Read the model definition and answer for the solid it produces. Units are mm, in the model's axes. A direction names the side the tool comes from. Round coordinates to 2 decimals unless told otherwise and drop trailing zeros. Write each loop counter-clockwise with the first axis right and the second up, starting at its lowest first coordinate (ties: lowest second). Pieces come first, ordered by that corner, then holes. Notation, with made-up numbers: (88.25, -19) - (100.25, -19) arc R22 cw to (100.25, 19) - close; hole circle Ø6 at (-29.5, -22). An arc over 180 degrees is marked (long way). Answer as CSV lines item,"result". Start each with the question number.
1) Consider line 1 along X through (y, z) = (8, 2.85); line 2 along Y through (x, z) = (-43, 1.35); line 3 along Z through (x, y) = (-38.75, -10). Determine where each line is inside the solid, lowest interval first.
2) Which of the six approach directions +Z, -Z, +X, -X, +Y, -Y give full straight-line access (tool end or side, diameter ignored) to faces 3 (the cylindrical face through (45.3, 9.2, 1.4)), 4 (the flat face through (-37.54, -10, 2)), 5 (the flat face through (-43.04, -9, 3)), 6 (the flat face through (-1, 0, 4))?
3) Find section A-A on y = -10. Determine the outline of the cut face in (x, z), then the cut area to 3 significant figures.
4) For a pull along Y with two mould halves and no side action, classify faces 1 (the flat face through (-47.54, 0, 2)), 2 (the flat face through (-40.04, 11, 3)) as +Y half, -Y half, draft (parallel to the pull), parting line (faces both ways), or undercut.
5) Each of these flat-tipped pins is pushed along its axis until it touches: pin 1 (1.5 mm diameter, centred on x = -42, z = 2.5, fed in from -Y); pin 2 (1.2 mm diameter, centred on y = -10, z = 2, fed in from -X); pin 3 (1.6 mm diameter, centred on y = 10, z = 2, fed in from +X). Where does it stop, or does it pass through?
from build123d import *

# Parameters (mm, degrees)
ESQUISSE1_W             = 95.08
ESQUISSE1_H             = 33.02
ESQUISSE1_W_2           = 3
ESQUISSE1_H_2           = 6
BOSS_EXTRU_1_DEPTH      = 4
CONG_1_R                = 3
ESQUISSE4_R             = 1
ENL_V_MAT_EXTRU_2_DEPTH = 10
ENL_V_START             = -10
ESQUISSE5_R             = 1
ENL_V_MAT_EXTRU_3_DEPTH = 10


with BuildPart() as part:
    # Esquisse1 → Boss.-Extru.1 (new body)
    with BuildSketch(Plane.XY):
        Rectangle(ESQUISSE1_W, ESQUISSE1_H)
        with Locations((-41.54, -10)):
            Rectangle(ESQUISSE1_W_2, ESQUISSE1_H_2, mode=Mode.SUBTRACT)
        with Locations((-41.54, 10)):
            Rectangle(ESQUISSE1_W_2, ESQUISSE1_H_2, mode=Mode.SUBTRACT)
        with Locations((41.54, -10)):
            Rectangle(ESQUISSE1_W_2, ESQUISSE1_H_2, mode=Mode.SUBTRACT)
        with Locations((41.54, 10)):
            Rectangle(ESQUISSE1_W_2, ESQUISSE1_H_2, mode=Mode.SUBTRACT)
    extrude(amount=BOSS_EXTRU_1_DEPTH)

    # Congé1
    cong_1_edges = [part.edges().sort_by_distance(p)[0] for p in [
        (0, -16.51, 4),
        (0, 16.51, 4),
    ]]
    fillet(cong_1_edges, radius=CONG_1_R)

    # Esquisse4 → Enlèv. mat.-Extru.2 (cut)
    with BuildSketch(Plane(origin=(47.54, 0, 0), x_dir=(0, 0, -1), z_dir=(1, 0, 0))):
        with Locations(Location((-2, 10, 0), (0, 0, 90))):
            Circle(ESQUISSE4_R)
        with Locations(Location((-2, -10, 0), (0, 0, 90))):
            Circle(ESQUISSE4_R)
    extrude(amount=-ENL_V_MAT_EXTRU_2_DEPTH, mode=Mode.SUBTRACT)

    # Esquisse5 → Enlèv. mat.-Extru.3 (cut)
    with BuildSketch(Plane.ZY.offset(47.54).offset(ENL_V_START)):
        with Locations(Location((2, 10, 0), (0, 0, 90))):
            Circle(ESQUISSE5_R)
        with Locations(Location((2, -10, 0), (0, 0, 90))):
            Circle(ESQUISSE5_R)
    extrude(amount=ENL_V_MAT_EXTRU_3_DEPTH, mode=Mode.SUBTRACT)


solid = part.part
Check values:
1,line 1,"x = -47.54 to -43.04, -40.04 to 40.04, 43.04 to 47.54"
1,line 2,"y = -16.49 to -13, -7 to 7, 13 to 16.49"
1,line 3,"z = 0 to 1, 3 to 4"
2,face 3,"+X"
2,face 4,"-X"
2,face 5,"+Z, -Z"
2,face 6,"+Z, +X, -X, +Y, -Y"
3,outline,"(-47.54, 0) - (-43.04, 0) - (-43.04, 1) - (-47.54, 1) - close; (-47.54, 3) - (-43.04, 3) - (-43.04, 4) - (-47.54, 4) - close; (-40.04, 0) - (40.04, 0) - (40.04, 1) - (37.54, 1) - (37.54, 3) - (40.04, 3) - (40.04, 4) - (-40.04, 4) - (-40.04, 3) - (-37.54, 3) - (-37.54, 1) - (-40.04, 1) - close; (43.04, 0) - (47.54, 0) - (47.54, 1) - (43.04, 1) - close; (43.04, 3) - (47.54, 3) - (47.54, 4) - (43.04, 4) - close"
3,area,"328 mm^2"
4,face 1,"draft"
4,face 2,"undercut"
5,pin 1,"stops at y = -16.41"
5,pin 2,"stops at x = -37.54"
5,pin 3,"stops at x = 37.54"
